from build123d import *

# Parameters (mm, degrees)
F0_R     = 14.7784
F0_R_2   = 1.778
F1_DEPTH = 4.318
F2_R     = 3.81
F3_DEPTH = 36.83


with BuildPart() as f1:
    # F0 (on Top) → F1 (new body)
    with BuildSketch(Plane.XY):
        Circle(F0_R)
        with Locations((0, -9.779)):
            Circle(F0_R_2, mode=Mode.SUBTRACT)
        with Locations((0, 9.779)):
            Circle(F0_R_2, mode=Mode.SUBTRACT)
    extrude(amount=F1_DEPTH)

    # F2 (on face) → F3 (join)
    with BuildSketch(Plane.XY.offset(4.318)):
        Circle(F2_R)
    extrude(amount=F3_DEPTH)


solid = f1.part
Build history of the part. All positions in model axes, mm. A direction names the side the tool comes from. Give positions to 0.01 mm unless a question says otherwise; leave off trailing zeros. Order: outer loops, then holes, each group sorted by start corner. A loop starts at its lowest first (then second) coordinate and runs counter-clockwise, first axis right, second up. Notation, with made-up numbers: M 37.5,87.5 L 69.5,87.5 A19 ccw 69.5,107.5 Z; hole C -11.75,5 d11. An arc over 180 degrees is marked long. Use one line per item in the form item = value.
1) Drop flat-ended pins along their axis: pin 1 (10 mm diameter, centred on x = -6, z = 16.5, fed in from +Y); pin 2 (5 mm diameter, centred on x = -3, z = 9, fed in from -Y); pin 3 (5 mm diameter, centred on x = 2.5, z = 9.5, fed in from +Y). Give the stop position or say it passes through.
Calculated:
pin_1 = 3.68
pin_2 = -3.78
pin_3 = 3.81
2) Saw through at A-A (x = 0). Give the cut face in (y, z).
Calculated:
outline = M -14.78,0 L -11.56,0 L -11.56,4.32 L -14.78,4.32 Z; M -8,0 L 8,0 L 8,4.32 L 3.81,4.32 L 3.81,41.15 L -3.81,41.15 L -3.81,4.32 L -8,4.32 Z; M 11.56,0 L 14.78,0 L 14.78,4.32 L 11.56,4.32 Z
3) Two-plate mould, pull along Y, no slides. Class faces 3 (the face through (-0.385, -11.515, 2.129)), 4 (the face through (0, 0, 41.148)), 5 (the face through (7.945, 12.461, 2.129)): released by +Y, released by -Y, zero draft, split by the parting line, or undercut.
Calculated:
face_3 = undercut
face_4 = zero draft
face_5 = split by the parting line
4) Saw through at B-B (y = 0). Give the cut face in (x, z), plus the area to 3 significant figures.
Calculated:
outline = M -14.78,0 L 14.78,0 L 14.78,4.32 L 3.81,4.32 L 3.81,41.15 L -3.81,41.15 L -3.81,4.32 L -14.78,4.32 Z
area = 408 mm2
5) Tool access for faces 1 (the face through (3, -3, 4.318)), 2 (the face through (0, 0, 0)): list every direction of +Z, -Z, +X, -X, +Y, -Y with a clear straight run to the whole face (end or side of a thin tool).
Calculated:
face_1 = +Z
face_2 = -Z, +X, -X, +Y, -Y
6) Saw through at D-D (x = -10.5). Give the cut face in (y, z).
Calculated:
outline = M -10.4,0 L 10.4,0 L 10.4,4.32 L -10.4,4.32 Z
7) Probe probe 1 along Y at (x, z) = (0, 1.3); probe 2 along Z at (x, y) = (2, 10.25); probe 3 along Y at (x, z) = (-0.25, 39.5). List the from-to ranges inside material, lowest first.
Calculated:
probe_1 = -14.78 to -11.56, -8 to 8, 11.56 to 14.78
probe_2 = 0 to 4.32
probe_3 = -3.8 to 3.8
8) Saw through at C-C (z = 14). Give the cut face in (x, y).
Calculated:
outline = C 0,0 d7.62
